Drawing for the job (mm, zero at the part's lowest x, y, z). A direction names the side the tool comes from. Coordinates: 2 decimals unless noted, no trailing zeros. Write each loop counter-clockwise with the first axis right and the second up, starting at its lowest first coordinate (ties: lowest second). Pieces come first, ordered by that corner, then holes. Notation, with made-up numbers: (-16.75, -2.5) -> (4.25, -2.5) arc R31 ccw to (4.25, 26.5) -> close; hole circle Ø1 at (25, -35). An arc over 180 degrees is marked (long way). Write item = value, one per line. Start each with the question number.
Q1. Pin check, flat tips, straight feed: P1, Ø9, axis at x = 45, z = 23.5, coming from the +Y side; P2, Ø4, axis at x = 6, z = 23, coming from the -Y side; P3, Ø6.5, axis at x = 44.5, z = 11.5, coming from the +Y side; P4, Ø2, axis at y = 31.5, z = 16.5, coming from the -X side. Stop position of each tip, or through.
Q2. Pull direction Z, two halves, no side cores. Call the marked faces 1, 2 and 3: released by +Z, released by -Z, zero draft, split by the parting line, or undercut.
Q3. Probe line 1 (Z direction, x = 44, y = 24.6); line 2 (X direction, y = 10.5, z = 23); line 3 (Z direction, x = 6, y = 18). List the from-to ranges inside material, lowest first.
Q4. Tool access for the marked faces 4, 5 and 6: list every direction of +Z, -Z, +X, -X, +Y, -Y with a clear straight run to the whole face (end or side of a thin tool).
Q5. Band-saw the part on B-B, the plane z = 12. Give the number of separate pieces and of enclosed holes in the cut face, plus the area to 3 significant figures.
Q6. Band-saw the part on C-C, the plane x = 44. List the corners of the cut face in (y, z).
Q7. Band-saw the part on D-D, the plane y = 3.5. List the corners of the cut face in (x, z), plus the area to 3 significant figures.
Q8. Band-saw the part on A-A, the plane y = 20. List the corners of the cut face in (x, z), plus the area to 3 significant figures.
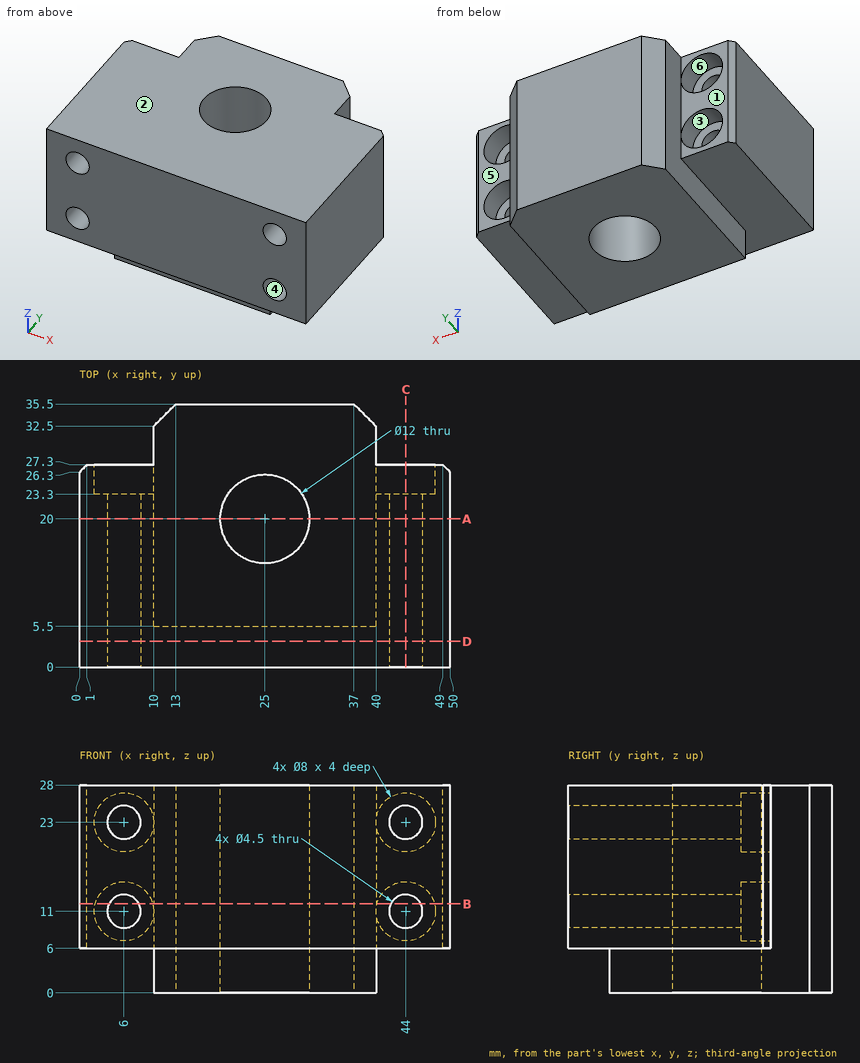
Ans:
q1.P1 = 27.3
q1.P2 = through
q1.P3 = 23.3
q1.P4 = 10
q2.face_1 = zero draft
q2.face_2 = released by +Z
q2.face_3 = undercut
q3.line_1 = 6 to 7, 15 to 19, 27 to 28
q3.line_2 = 0 to 3.75, 8.25 to 41.75, 46.25 to 50
q3.line_3 = 6 to 8.75, 13.25 to 20.75, 25.25 to 28
q4.face_4 = +Y, -Y
q4.face_5 = +Z, -Z, +X, +Y
q4.face_6 = +Y
q5.separate_pieces = 3
q5.enclosed_holes = 1
q5.area = 1,240 mm2
q6.outline = (0, 6) -> (27.3, 6) -> (27.3, 7) -> (23.3, 7) -> (23.3, 8.75) -> (0, 8.75) -> close; (0, 13.25) -> (23.3, 13.25) -> (23.3, 15) -> (27.3, 15) -> (27.3, 19) -> (23.3, 19) -> (23.3, 20.75) -> (0, 20.75) -> close; (0, 25.25) -> (23.3, 25.25) -> (23.3, 27) -> (27.3, 27) -> (27.3, 28) -> (0, 28) -> close
q7.outline = (0, 6) -> (50, 6) -> (50, 28) -> (0, 28) -> close; hole circle Ø4.5 at (6, 11); hole circle Ø4.5 at (6, 23); hole circle Ø4.5 at (44, 11); hole circle Ø4.5 at (44, 23)
q7.area = 1,040 mm2
q8.outline = (0, 6) -> (10, 6) -> (10, 0) -> (19, 0) -> (19, 28) -> (0, 28) -> close; (31, 0) -> (40, 0) -> (40, 6) -> (50, 6) -> (50, 28) -> (31, 28) -> close; hole circle Ø4.5 at (6, 11); hole circle Ø4.5 at (6, 23); hole circle Ø4.5 at (44, 11); hole circle Ø4.5 at (44, 23)
q8.area = 880 mm2
